Autodesk Inventor part; units mm, degrees
ref_plane "YZ Plane" through (0, 0, 0) normal (1, 0, 0) x (0, 1, 0)
ref_plane "XZ Plane" through (0, 0, 0) normal (0, 1, 0) x (-1, 0, 0)
ref_plane "XY Plane" through (0, 0, 0) normal (0, 0, 1) x (1, 0, 0)
sketch "Esquisse2" plane through (0, 0, 0) normal (0, 1, 0) x (-1, 0, 0)
  line L0 (-7, 113) -> (7, 113)
  line L1 (7, 113) -> (7, -113)
  line L2 (7, -113) -> (-7, -113)
  line L3 (-7, -113) -> (-7, 113)
  line L4 (-7, 113) -> (7, -113) construction
  line L5 (7, 113) -> (-7, -113) construction
  point P0 (0, 0)
  dimension "d0" = 226
  dimension "d1" = 14
extrude "Extrusion1" add sketch "Esquisse2" along normal blind 1
sketch "Esquisse3" plane through (0, 1, 0) normal (0, 1, 0) x (1, 0, 0)
  line L0 (7, 113) -> (-7, 113)
  line L1 (-7, -113) -> (7, -113)
  point P0 (0, 0)
  point P1 (0, -107)
  point P2 (0, 108)
  dimension "d4" = 5
  dimension "d14" = 215
hole "Perçage1" at (0, 1, 107) at (0, 1, -108) direction (0, -1, 0) diameter 4.5 end through all
sketch "Esquisse4" plane through (0, 1, 0) normal (0, 1, 0) x (1, 0, 0)
  line L0 (0, 3) -> (0, -53) construction
  line L1 (-2.75, 3) -> (-2.75, -53)
  line L2 (2.75, -53) -> (2.75, 3)
  arc A0 (2.75, 3) -> (-2.75, 3) centre (0, 3) ccw
  arc A1 (-2.75, -53) -> (2.75, -53) centre (0, -53) ccw
  line L3 (7, 113) -> (-7, 113)
  line L4 (-7, -113) -> (7, -113)
  point P0 (0, 0)
  point P1 (0, -25)
  dimension "d15" = 56
  dimension "d17" = 5.5
  dimension "d21" = 60
extrude "Extrusion2" cut sketch "Esquisse4" against normal up to surface (1 mm away)
properties part number "support_lateral" material "Aluminium 6061"
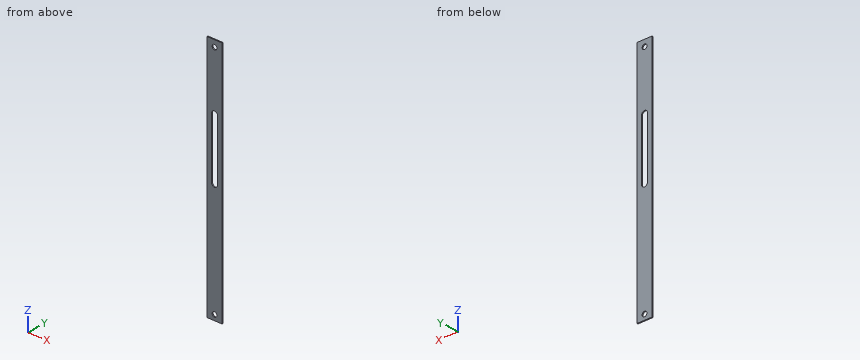
Verification items for the finished model (mm, model axes). Coordinates: 2 decimals unless noted, no trailing zeros. Order: outer loops, then holes, each group sorted by start corner. A loop starts at its lowest first (then second) coordinate and runs counter-clockwise, first axis right, second up.
Item 1: Section check B-B, the plane z = -108. Enter the section's corners in (x, y).
Filled in:
outline: (-7, 0) - (-2.25, 0) - (-2.25, 1) - (-7, 1) - close; (2.25, 0) - (7, 0) - (7, 1) - (2.25, 1) - close
Item 2: Section check A-A, the plane x = 0. Enter the section's corners in (y, z), then the cut area to 4 significant figures.
Filled in:
outline: (0, -113) - (1, -113) - (1, -110.25) - (0, -110.25) - close; (0, -105.75) - (1, -105.75) - (1, -5.75) - (0, -5.75) - close; (0, 55.75) - (1, 55.75) - (1, 104.75) - (0, 104.75) - close; (0, 109.25) - (1, 109.25) - (1, 113) - (0, 113) - close
area: 155.5 mm2
Item 3: Section check C-C, the plane y = 0.8. Enter the section's corners in (x, z), then the cut area to 3 significant figures.
Filled in:
outline: (-7, -113) - (7, -113) - (7, 113) - (-7, 113) - close; hole (-2.75, -3) arc R2.75 ccw to (2.75, -3) - (2.75, 53) arc R2.75 ccw to (-2.75, 53) - close; hole circle Ø4.5 at (0, -108); hole circle Ø4.5 at (0, 107)
area: 2,800 mm2
Item 4: Material ranges on L1, parallel to Z at x = 0, y = 0.45; L2, parallel to X at y = 0.45, z = -0.5; L3, parallel to X at y = 0.75, z = -108, recorded low to high.
Filled in:
L1: z = -113 to -110.25, -105.75 to -5.75, 55.75 to 104.75, 109.25 to 113
L2: x = -7 to -2.75, 2.75 to 7
L3: x = -7 to -2.25, 2.25 to 7
